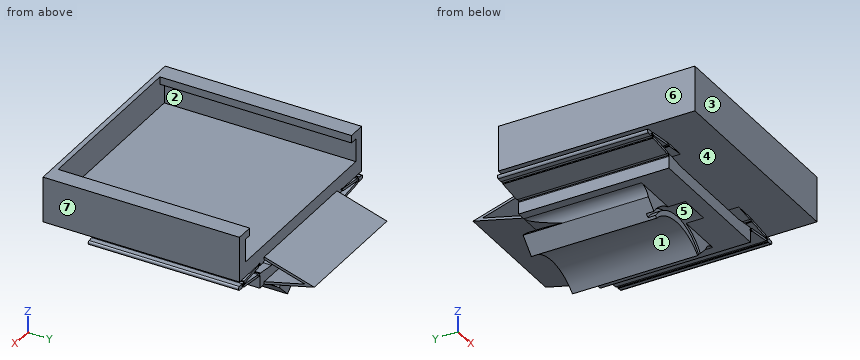
from build123d import *

# Parameters (mm, degrees)
F1_DEPTH      = 76.5
F3_DEPTH      = 60
F4_W          = 84
F4_H          = 2
F5_DEPTH      = 12.2
F5_DEPTH_BACK = 6
F7_DEPTH      = 25
F7_DEPTH_BACK = 25
F8_W          = 50
F8_H          = 8
F9_ANGLE_BACK = 45
F9_ANGLE      = 90
F10_T4_DEPTH  = 68.2385540506
F10_T9_DEPTH  = 68.2385540506
F11_W         = 5
F11_H         = 1.5
F14_DEPTH     = 60
F15_F1_R      = 0.75
F15_F2_R      = 0.75


# Not quite as in the source:
# - a fillet or chamfer that OpenCascade refuses, or shapes differently, is made with other operations: its cross-section is extruded or revolved along the edge and cut away or added


with BuildPart() as f1:
    # F0 (on Front) → F1 (new body)
    with BuildSketch(Plane.XZ):
        Polygon((-35, 9.2), (-35, 12.2), (-42, 12.2), (-42, -6), (0, -6), (42, -6), (42, 12.2), (35, 12.2), (35, 9.2), (38, 9.2), (38, 0), (0, 0), (-38, 0), (-38, 9.2), align=None)
    extrude(amount=F1_DEPTH)

    # F2 (on Front) → F3 (join)
    with BuildSketch(Plane.XZ):
        Polygon((-40, -8.5), (-20, -6), (-28.0622577483, -6), (-48.0622577483, -8.5), (-28.0622577483, -11), (-28.0622577483, -16), (0, -16), (28.0622577483, -16), (28.0622577483, -11), (48.0622577483, -8.5), (28.0622577483, -6), (20, -6), (40, -8.5), (20, -11), (0, -11), (-20, -11), align=None)
    extrude(amount=F3_DEPTH)

    # F4 (on face) → F5 (join, two sides)
    with BuildSketch(Plane.XY) as f5_sk:
        with Locations((0, -77.5)):
            Rectangle(F4_W, F4_H)
    extrude(amount=F5_DEPTH)
    extrude(f5_sk.sketch, amount=-F5_DEPTH_BACK)

    # F6 (on Right) → F7 (join, two sides)
    with BuildSketch(Plane.YZ) as f7_sk:
        Polygon((0, -14.9692235936), (0, -16), (20, -11), (0, -4.9240960793), (0, -5.9692235936), (16.2514952539, -10.9063497801), align=None)
        Polygon((-20, -11), (0, -16), (0, -14.9692235936), (-16.2514952539, -10.9063497801), (0, -5.9692235936), (0, -4.9240960793), align=None)
    extrude(amount=F7_DEPTH)
    extrude(f7_sk.sketch, amount=-F7_DEPTH_BACK)

    # F8 (on Right) → F9 (revolve)
    with BuildSketch(Plane.YZ, mode=Mode.PRIVATE) as f9_sk:
        with Locations((-22, -15)):
            Rectangle(F8_W, F8_H)
    revolve(f9_sk.sketch.rotate(Axis((0, -22, -39), (0, 1, 0)), -F9_ANGLE_BACK), axis=Axis((0, -22, -39), (0, 1, 0)), revolution_arc=F9_ANGLE)

    # F10: fillet of radius 5 on 2 edges, made by hand


with BuildPart() as f10_tool2:
    # F10_s3 → F10_t4 (new body)
    with BuildSketch(Plane.XZ.offset(-21.2385540506)):
        with BuildLine():
            ThreePointArc((-19.7989898732, -19.2010101268), (-21.6352675362, -16.8772006254), (-24.4641410429, -16))
            Line((-24.4641410429, -16), (-15.9687194227, -16))
            ThreePointArc((-15.9687194227, -16), (-17.9553299476, -17.5149790209), (-19.7989898732, -19.2010101268))
        make_face()
    extrude(amount=F10_T4_DEPTH)

    split(bisect_by=Plane(origin=(0, 3.7647058824, -15.0588235294), x_dir=(1, 0, 0), z_dir=(0, -0.242535625, 0.9701425001)), keep=Keep.TOP)


with BuildPart() as f1_1:
    add(f1.part)

    # F10_t1: union F10_tool2
    add(f10_tool2.part)


with BuildPart() as f10_tool7:
    # F10_s8 → F10_t9 (new body)
    with BuildSketch(Plane.XZ.offset(-21.2385540506)):
        with BuildLine():
            ThreePointArc((19.7989898732, -19.2010101268), (21.6352675362, -16.8772006254), (24.4641410429, -16))
            Line((24.4641410429, -16), (15.9687194227, -16))
            ThreePointArc((15.9687194227, -16), (17.9553299476, -17.5149790209), (19.7989898732, -19.2010101268))
        make_face()
    extrude(amount=F10_T9_DEPTH)

    split(bisect_by=Plane(origin=(0, 3.7647058824, -15.0588235294), x_dir=(1, 0, 0), z_dir=(0, -0.242535625, 0.9701425001)), keep=Keep.TOP)


with BuildPart() as f1_2:
    add(f1_1.part)

    # F10_t6: union F10_tool7
    add(f10_tool7.part)

    # F11 (on Right) → F12 (revolve, cut)
    with BuildSketch(Plane.YZ):
        with Locations((-51.5, -15.75)):
            Rectangle(F11_W, F11_H)
        with Locations((-46.5, -15.75)):
            Rectangle(F11_W, F11_H)
    revolve(axis=Axis((0, -22, -34.8578643763), (0, 1, 0)), mode=Mode.SUBTRACT)

    # F13 (on face) → F14 (cut, through all)
    with BuildSketch(Plane.XZ.offset(60)):
        with BuildLine():
            Line((38.9456393414, -8.8837402215), (40, -8.75))
            ThreePointArc((40, -8.75), (40.25, -8.5), (40, -8.25))
            Line((40, -8.25), (39.0077436029, -8.1257935491))
            ThreePointArc((39.0077436029, -8.1257935491), (38.8060744602, -8.1623581433), (38.6995205721, -8.3374400715))
            Line((38.6995205721, -8.3374400715), (38.6661107322, -8.6047187912))
            ThreePointArc((38.6661107322, -8.6047187912), (38.737564097, -8.8126646153), (38.9456393414, -8.8837402215))
        make_face()
        with BuildLine():
            Line((39.0699789435, -7.627910704), (40.0622568202, -7.7519454386))
            ThreePointArc((40.0622568202, -7.7519454386), (40.341334973, -7.5348846531), (40.1242741875, -7.2558065003))
            Line((40.1242741875, -7.2558065003), (39.1319963108, -7.1317717657))
            ThreePointArc((39.1319963108, -7.1317717657), (38.8529181579, -7.3488325512), (39.0699789435, -7.627910704))
        make_face()
        with BuildLine():
            Line((29.054535625, -5.8740347346), (28.0622577483, -5.75))
            ThreePointArc((28.0622577483, -5.75), (27.8141882791, -5.9689913164), (28.0007192868, -6.2423076923))
            Line((28.0007192868, -6.2423076923), (28.9929971635, -6.3663424269))
            ThreePointArc((28.9929971635, -6.3663424269), (29.2699202404, -6.1509578115), (29.054535625, -5.8740347346))
        make_face()
        with BuildLine():
            Line((28.9307403433, -6.8643969883), (27.9384624666, -6.7403622537))
            ThreePointArc((27.9384624666, -6.7403622537), (27.6593843138, -6.9574230392), (27.8764450993, -7.236501192))
            Line((27.8764450993, -7.236501192), (28.868722976, -7.3605359266))
            ThreePointArc((28.868722976, -7.3605359266), (29.1478011288, -7.1434751411), (28.9307403433, -6.8643969883))
        make_face()
        with BuildLine():
            ThreePointArc((39.0699789435, -9.372089296), (38.8529181579, -9.6511674488), (39.1319963108, -9.8682282343))
            Line((39.1319963108, -9.8682282343), (40.1242741875, -9.7441934997))
            ThreePointArc((40.1242741875, -9.7441934997), (40.341334973, -9.4651153469), (40.0622568202, -9.2480545614))
            Line((40.0622568202, -9.2480545614), (39.0699789435, -9.372089296))
        make_face()
        with BuildLine():
            Line((27.9384624666, -10.2596377463), (28.9307403433, -10.1356030117))
            ThreePointArc((28.9307403433, -10.1356030117), (29.1478011288, -9.8565248589), (28.868722976, -9.6394640734))
            Line((28.868722976, -9.6394640734), (27.8764450993, -9.763498808))
            ThreePointArc((27.8764450993, -9.763498808), (27.6593843138, -10.0425769608), (27.9384624666, -10.2596377463))
        make_face()
        with BuildLine():
            ThreePointArc((28.0007192868, -10.7576923077), (27.8141882791, -11.0310086836), (28.0622577483, -11.25))
            Line((28.0622577483, -11.25), (29.054535625, -11.1259652654))
            ThreePointArc((29.054535625, -11.1259652654), (29.2699202404, -10.8490421885), (28.9929971635, -10.6336575731))
            Line((28.9929971635, -10.6336575731), (28.0007192868, -10.7576923077))
        make_face()
        with BuildLine():
            Line((-38.6661107322, -8.6047187912), (-38.6995205721, -8.3374400715))
            ThreePointArc((-38.6995205721, -8.3374400715), (-38.8060744602, -8.1623581433), (-39.0077436029, -8.1257935491))
            Line((-39.0077436029, -8.1257935491), (-40, -8.25))
            ThreePointArc((-40, -8.25), (-40.25, -8.5), (-40, -8.75))
            Line((-40, -8.75), (-38.9456393414, -8.8837402215))
            ThreePointArc((-38.9456393414, -8.8837402215), (-38.737564097, -8.8126646153), (-38.6661107322, -8.6047187912))
        make_face()
        with BuildLine():
            Line((-40.0622568202, -7.7519454386), (-39.0699789435, -7.627910704))
            ThreePointArc((-39.0699789435, -7.627910704), (-38.8529181579, -7.3488325512), (-39.1319963108, -7.1317717657))
            Line((-39.1319963108, -7.1317717657), (-40.1242741875, -7.2558065003))
            ThreePointArc((-40.1242741875, -7.2558065003), (-40.341334973, -7.5348846531), (-40.0622568202, -7.7519454386))
        make_face()
        with BuildLine():
            ThreePointArc((-39.1319963108, -9.8682282343), (-38.8529181579, -9.6511674488), (-39.0699789435, -9.372089296))
            Line((-39.0699789435, -9.372089296), (-40.0622568202, -9.2480545614))
            ThreePointArc((-40.0622568202, -9.2480545614), (-40.341334973, -9.4651153469), (-40.1242741875, -9.7441934997))
            Line((-40.1242741875, -9.7441934997), (-39.1319963108, -9.8682282343))
        make_face()
        with BuildLine():
            ThreePointArc((-28.0007192868, -6.2423076923), (-27.8141882791, -5.9689913164), (-28.0622577483, -5.75))
            Line((-28.0622577483, -5.75), (-29.054535625, -5.8740347346))
            ThreePointArc((-29.054535625, -5.8740347346), (-29.2699202404, -6.1509578115), (-28.9929971635, -6.3663424269))
            Line((-28.9929971635, -6.3663424269), (-28.0007192868, -6.2423076923))
        make_face()
        with BuildLine():
            ThreePointArc((-27.9384624666, -10.2596377463), (-27.6593843138, -10.0425769608), (-27.8764450993, -9.763498808))
            Line((-27.8764450993, -9.763498808), (-28.868722976, -9.6394640734))
            ThreePointArc((-28.868722976, -9.6394640734), (-29.1478011288, -9.8565248589), (-28.9307403433, -10.1356030117))
            Line((-28.9307403433, -10.1356030117), (-27.9384624666, -10.2596377463))
        make_face()
        with BuildLine():
            ThreePointArc((-28.0622577483, -11.25), (-27.8141882791, -11.0310086836), (-28.0007192868, -10.7576923077))
            Line((-28.0007192868, -10.7576923077), (-28.9929971635, -10.6336575731))
            ThreePointArc((-28.9929971635, -10.6336575731), (-29.2699202404, -10.8490421885), (-29.054535625, -11.1259652654))
            Line((-29.054535625, -11.1259652654), (-28.0622577483, -11.25))
        make_face()
        with BuildLine():
            ThreePointArc((-27.8764450993, -7.236501192), (-27.6593843138, -6.9574230392), (-27.9384624666, -6.7403622537))
            Line((-27.9384624666, -6.7403622537), (-28.9307403433, -6.8643969883))
            ThreePointArc((-28.9307403433, -6.8643969883), (-29.1478011288, -7.1434751411), (-28.868722976, -7.3605359266))
            Line((-28.868722976, -7.3605359266), (-27.8764450993, -7.236501192))
        make_face()
    extrude(amount=-F14_DEPTH, mode=Mode.SUBTRACT)

    # F15: fillet of radius 0.75 on 2 edges, made by hand

    # F15_f1
    f15_f1_edges = [f1_2.edges().sort_by_distance(p)[0] for p in [
        (-48.0622577483, -30, -8.5),
    ]]
    fillet(f15_f1_edges, radius=F15_F1_R)

    # F15_f2
    f15_f2_edges = [f1_2.edges().sort_by_distance(p)[0] for p in [
        (48.0622577483, -30, -8.5),
    ]]
    fillet(f15_f2_edges, radius=F15_F2_R)


solid = f1_2.part
Work out the finished part from the listing and answer in its coordinate system (mm). Face numbers are marked on the shaded views. A direction names the side the tool comes from. Give positions to 0.01 mm unless a question says otherwise; leave off trailing zeros. Loops run counter-clockwise (first coordinate to the right, second up) from the corner with the lowest first, then second, coordinate; pieces in that order, holes last. Notation, with made-up numbers: M -4,-24.5 L 30,-24.5 A19 cw 30,-6.5 Z; hole C 54.5,86.5 d6. An arc over 180 degrees is marked long. Use CSV: the item, a comma, the result in double quotes.
1) Find section C-C on y = -8. Give the number of separate pieces and of enclosed holes in the cut face, plus the area to 3 significant figures.
Answer:
separate pieces,"2"
enclosed holes,"1"
area,"1,230 mm^2"
2) Consider L1, parallel to Z at x = -32, y = -17; L2, parallel to Z at x = 21, y = -5 (3 decimals); L3, parallel to Z at x = -35.5, y = -12.5. Determine where each line is inside the solid, lowest interval first.
Answer:
L1,"-10.51 to -9.5, -7.5 to -6.49, -6 to 0"
L2,"-17.25 to -10.875, -7.488 to -6.443, -6.125 to 0"
L3,"-10.07 to -9.06, -7.94 to -6.93, -6 to 0, 9.2 to 12.2"
3) Find section B-B on z = -2.5. Write down the section's boundary in (x, y), plus the area to 3 significant figures.
Answer:
outline,"M -42,-78.5 L 42,-78.5 L 42,0 L -42,0 Z"
area,"6,590 mm^2"
4) Determine the mould class of the marked faces 1, 2 and 3 for opening direction Z: released by +Z, released by -Z, zero draft, split by the parting line, or undercut.
Answer:
face 1,"released by -Z"
face 2,"undercut"
face 3,"zero draft"
5) Which of the six approach directions +Z, -Z, +X, -X, +Y, -Y give full straight-line access (tool end or side, diameter ignored) to the marked faces 4, 5, 6 and 7?
Answer:
face 4,"-Y"
face 5,"none"
face 6,"+Z, -X, +Y, -Y"
face 7,"+Z, +X, +Y, -Y"
6) Given P1, Ø3, axis at x = 31.5, y = -8.5, coming from the +Z side; P2, Ø5.5, axis at y = 8.5, z = -9, coming from the -X side; P3, Ø8, axis at y = -50.5, z = -4, coming from the +X side, each flat-ended and moving along its own axis, determine where each tip first touches the part or whether it passes through.
Answer:
P1,"z = 0"
P2,"x = -25"
P3,"x = 42.57"
